Could you check a few things on this model? Use its own coordinates, in mm. A direction names the side the tool comes from. Coordinates: 2 decimals unless noted, no trailing zeros. Loops run counter-clockwise (first coordinate to the right, second up) from the corner with the lowest first, then second, coordinate; pieces in that order, holes last. Notation, with made-up numbers: (75, 30.5) - (118, 30.5) arc R37 cw to (118, 66.5) - close; hole circle Ø10 at (70.5, 85). An arc over 180 degrees is marked (long way). One line per question, with ' | ' between items. Start each with the question number.
1. I want a section at D-D, the plane z = -885.5. Write out the boundary of the cut face in (x, y), then the cut area to 3 significant figures.
2. I want a section at A-A, the plane z = -1354.5. Write out the boundary of the cut face in (x, y), then the cut area to 3 significant figures.
3. I want a section at C-C, the plane y = 406. Write out the boundary of the cut face in (x, z).
4. We'd pull the mould along Z, two halves only. Please class faces 6 (the cylindrical face through (1744.576, 593, -552.654)), 7 (the flat face through (1774, 25, 12.024)), 8 (the flat face through (1845.838, 1149, -1026)): pulls with the +Z half, pulls with the -Z half, needs draft (parallel to the pull), parting line crosses it, or undercut.
5. I'm going to push flat-ended pins straight in: P1, Ø6, axis at x = 1741.5, y = 515.5, coming from the -Z side; P2, Ø5, axis at x = 1789.5, y = 759, coming from the +Z side; P3, Ø8, axis at x = 1728.5, y = 779, coming from the -Z side. Where does each tip first touch, or does it pass through?
6. Please list where these lines run through material, in increasing order: L1, parallel to Y at x = 1736, z = -1112; L2, parallel to Z at x = 1747.5, y = 850.5; L3, parallel to Z at x = 1816.5, y = 1056. Write a range as [from, to].
7. Which directions (+Z, -Z, +X, -X, +Y, -Y) give clear straight access to the entire face, cutting with the end or side of a thin tool? Please do faces 1 (the flat face through (1704.162, 1149, -1050)), 2 (the cylindrical face through (1776.558, 1149.3, -1983.797)), 3 (the cylindrical face through (1777.198, 593, -1262.928)), 4 (the flat face through (1774, 0, -1053)), 5 (the cylindrical face through (1773.442, 1149.3, -92.155)).
8. I want a section at B-B, the plane x = 1775. Count the separate pieces of the cut face and the enclosed holes in it, then the cut area to 3 significant figures.
from build123d import *

# Parameters (mm, degrees)
SKETCH2_W               = 150
SKETCH2_H               = 2100
BOSS_EXTRUDE3_DEPTH     = 100
BOSS_EXTRUDE3_2_DEPTH   = 100
SKETCH3_R               = 50
BOSS_EXTRUDE4_DEPTH     = 1000
LPATTERN1_COUNT         = 6
LPATTERN1_PITCH         = 350
SKETCH5_R               = 50
BOSS_EXTRUDE5_DEPTH     = 1000
LPATTERN2_COUNT         = 6
LPATTERN2_PITCH         = 350
FILLET1_R               = 50
FILLET2_R               = 50
FILLET3_R               = 50
FILLET4_R               = 50
BOSS_EXTRUDE8_DEPTH     = 100
CUT_EXTRUDE1_DEPTH      = 2000
CUT_EXTRUDE1_DEPTH_BACK = 2000
SKETCH14_W              = 805.257541721
SKETCH14_H              = 2502.966116942


with BuildPart() as part:
    # Sketch2 → Boss-Extrude3 (new body)
    with BuildSketch(Plane(origin=(0, 0, 0), x_dir=(1, 0, 0), z_dir=(0, 1, 0))):
        with Locations((1775, 1037.975951904)):
            Rectangle(SKETCH2_W, SKETCH2_H)
    extrude(amount=BOSS_EXTRUDE3_DEPTH)

    # Sketch5 → Boss-Extrude5 (add)
    with BuildSketch(Plane(origin=(0, 100, 0), x_dir=(1, 0, 0), z_dir=(0, 1, 0))):
        with Locations(Location((1775, 1912.975951904, 0), (0, 0, 270))):
            Circle(SKETCH5_R)
    boss_extrude5 = extrude(amount=BOSS_EXTRUDE5_DEPTH)

    # LPattern2: Boss-Extrude5 ×6
    with Locations(*[(0, 0, i * LPATTERN2_PITCH) for i in range(1, LPATTERN2_COUNT)]):
        add(boss_extrude5)

    # Fillet3
    fillet3_edges = [part.edges().sort_by_distance(p)[0] for p in [
        (1775, 100, 12.024048096),
    ]]
    fillet(fillet3_edges, radius=FILLET3_R)

    # Fillet4
    fillet4_edges = [part.edges().sort_by_distance(p)[0] for p in [
        (1775, 100, -2087.975951904),
    ]]
    fillet(fillet4_edges, radius=FILLET4_R)



with BuildPart() as body_2:
    # Sketch2 → Boss-Extrude3 2 (new body)
    with BuildSketch(Plane(origin=(0, 0, 0), x_dir=(1, 0, 0), z_dir=(0, 1, 0))):
        with Locations((-1775, 1037.975951904)):
            Rectangle(SKETCH2_W, SKETCH2_H)
    extrude(amount=BOSS_EXTRUDE3_2_DEPTH)

    # Sketch3 → Boss-Extrude4 (add)
    with BuildSketch(Plane(origin=(0, 100, 0), x_dir=(1, 0, 0), z_dir=(0, 1, 0))):
        with Locations(Location((-1775, 162.975951904, 0), (0, 0, 90))):
            Circle(SKETCH3_R)
    boss_extrude4 = extrude(amount=BOSS_EXTRUDE4_DEPTH)

    # LPattern1: Boss-Extrude4 ×6
    with Locations(*[(0, 0, -i * LPATTERN1_PITCH) for i in range(1, LPATTERN1_COUNT)]):
        add(boss_extrude4)

    # Fillet1
    fillet1_edges = [body_2.edges().sort_by_distance(p)[0] for p in [
        (-1775, 100, -2087.975951904),
    ]]
    fillet(fillet1_edges, radius=FILLET1_R)

    # Fillet2
    fillet2_edges = [body_2.edges().sort_by_distance(p)[0] for p in [
        (-1775, 100, 12.024048096),
    ]]
    fillet(fillet2_edges, radius=FILLET2_R)


with BuildPart() as part_1:
    add(part.part)

    add(body_2.part)  # Boss-Extrude8 merges body 2
    # Sketch13 → Boss-Extrude8 (add)
    with BuildSketch(Plane(origin=(0, 1100, 0), x_dir=(1, 0, 0), z_dir=(0, 1, 0))):
        with BuildLine():
            Line((-1845.838339321, 162.975951904), (-1845.838339321, 1912.975951904))
            ThreePointArc((-1845.838339321, 1912.975951904), (-1775, 1983.814291225), (-1704.161660679, 1912.975951904))
            Line((-1704.161660679, 1912.975951904), (-1704.161660679, 162.975951904))
            ThreePointArc((-1704.161660679, 162.975951904), (-1775, 92.137612583), (-1845.838339321, 162.975951904))
        make_face()
        with BuildLine():
            Line((1845.838339321, 162.975951904), (1845.838339321, 1912.975951904))
            ThreePointArc((1845.838339321, 1912.975951904), (1775, 1983.814291225), (1704.161660679, 1912.975951904))
            Line((1704.161660679, 1912.975951904), (1704.161660679, 162.975951904))
            ThreePointArc((1704.161660679, 162.975951904), (1775, 92.137612583), (1845.838339321, 162.975951904))
        make_face()
    extrude(amount=BOSS_EXTRUDE8_DEPTH)

    # Sketch14 → Cut-Extrude1 (cut, two sides: drawn at the far end of the back side and taken through both)
    with BuildSketch(Plane(origin=(0, 1100, 0), x_dir=(1, 0, 0), z_dir=(0, 1, 0)).offset(-CUT_EXTRUDE1_DEPTH_BACK)):
        with Locations((-1496.523875696, 935.395373341)):
            Rectangle(SKETCH14_W, SKETCH14_H)
    extrude(amount=CUT_EXTRUDE1_DEPTH + CUT_EXTRUDE1_DEPTH_BACK, mode=Mode.SUBTRACT)


solid = part_1.part
Results are:
1) outline: (1700, 0) - (1850, 0) - (1850, 100) - (1819.64, 100) - (1819.64, 1100) - (1845.84, 1100) - (1845.84, 1200) - (1704.16, 1200) - (1704.16, 1100) - (1730.36, 1100) - (1730.36, 100) - (1700, 100) - close | area: 118,000 mm2
2) outline: (1700, 0) - (1850, 0) - (1850, 100) - (1700, 100) - close; (1704.16, 1100) - (1845.84, 1100) - (1845.84, 1200) - (1704.16, 1200) - close | area: 29,200 mm2
3) outline: circle Ø100 at (1775, -1912.98); circle Ø100 at (1775, -1562.98); circle Ø100 at (1775, -1212.98); circle Ø100 at (1775, -862.98); circle Ø100 at (1775, -512.98); circle Ø100 at (1775, -162.98)
4) face 6: undercut | face 7: pulls with the +Z half | face 8: needs draft
5) P1: stops at z = -1952.6 | P2: stops at z = -114.44 | P3: stops at z = -1939.32
6) L1: y = [0, 100], [1100, 1200] | L2: z = [-1954.73, -1871.22], [-1604.73, -1521.22], [-1254.73, -1171.22], [-904.73, -821.22], [-554.73, -471.22], [-204.73, -121.22] | L3: z = [-1940.86, -1885.09], [-1590.86, -1535.09], [-1240.86, -1185.09], [-890.86, -835.09], [-540.86, -485.09], [-190.86, -135.09]
7) face 1: +Z, -Z, -X, +Y | face 2: -Z, +Y | face 3: none | face 4: +Z, -Z, +X, -X, -Y | face 5: +Z, +Y
8) separate pieces: 1 | enclosed holes: 5 | area: 998,000 mm2
